```python
from build123d import *

# Parameters (mm, degrees)
F0_W      = 539.75
F0_H      = 53.975
F1_DEPTH  = 635
F2_W      = 482.854
F2_H      = 578.104
F3_DEPTH  = 25.4
F1_FACE_W = 539.75
F1_FACE_H = 635
F5_DEPTH  = 28.575


with BuildPart() as f1:
    # F0 (on Front) → F1 (new body)
    with BuildSketch(Plane.XZ):
        with Locations((269.875, 26.9875)):
            Rectangle(F0_W, F0_H)
    extrude(amount=-F1_DEPTH)

    # F2 (on face) → F3 (cut)
    with BuildSketch(Plane.XY.offset(53.975)):
        with Locations((269.875, 317.5)):
            Rectangle(F2_W, F2_H)
    extrude(amount=-F3_DEPTH, mode=Mode.SUBTRACT)


with BuildPart() as f5:
    # F1_face (on face) → F5 (new body)
    with BuildSketch(Plane(origin=(269.875, 317.5, 53.975), x_dir=(1, 0, 0), z_dir=(0, 0, 1))):
        Rectangle(F1_FACE_W, F1_FACE_H)
    extrude(amount=F5_DEPTH)


solid = f1.part
```
Source: CAD feature listing. Evaluate the final solid. Frame: model axes, mm. A direction names the side the tool comes from. Give positions to 0.01 mm unless a question says otherwise; leave off trailing zeros. Order: outer loops, then holes, each group sorted by start corner. A loop starts at its lowest first (then second) coordinate and runs counter-clockwise, first axis right, second up. Notation, with made-up numbers: (65.5, 77) -> (120.5, 77) arc R23 ccw to (120.5, 93) -> close; hole circle Ø4 at (38, 12). An arc over 180 degrees is marked (long way). Use a Markdown table: item, result.
Q1. Section C-C (x = 368). Return the cut outline in (y, z) (3 decimals).
A:
| item | result |
|---|---|
| outline | (0, 0) -> (635, 0) -> (635, 53.975) -> (606.552, 53.975) -> (606.552, 28.575) -> (28.448, 28.575) -> (28.448, 53.975) -> (0, 53.975) -> close |
Q2. Section B-B (z = 45.5). Return the cut outline in (x, y).
A:
| item | result |
|---|---|
| outline | (0, 0) -> (539.75, 0) -> (539.75, 635) -> (0, 635) -> close; hole (28.45, 28.45) -> (511.3, 28.45) -> (511.3, 606.55) -> (28.45, 606.55) -> close |
Q3. Pull-direction query (Y, two-part tool) for faces 3 (the face through (266, 606.552, 41)), 4 (the face through (0, 313, 27)), 5 (the face through (266, 0, 27)); classes: +Y half, -Y half, draft (parallel to the pull), parting line (faces both ways), or undercut.
A:
| item | result |
|---|---|
| face 3 | undercut |
| face 4 | draft |
| face 5 | -Y half |
Q4. First-contact query: P1, Ø5, axis at x = 267.5, z = 8.5, coming from the -Y side; P2, Ø4, axis at x = 195.5, y = 417.5, coming from the +Z side (3 decimals). Flat tips, straight axial feed; report the tip coordinate or a pass-through.
A:
| item | result |
|---|---|
| P1 | y = 0 |
| P2 | z = 28.575 |
Q5. Access query for faces 1 (the face through (266, 635, 27)), 2 (the face through (266, 28.448, 41)). Directions: +Z, -Z, +X, -X, +Y, -Y. A direction counts if a zero-diameter tool reaches every point of the face in a straight line with its end or side. Return the directions, or none.
A:
| item | result |
|---|---|
| face 1 | +Z, -Z, +X, -X, +Y |
| face 2 | +Z |
Q6. Section A-A (y = 242). Return the cut outline in (x, z) (3 decimals), and give its area (3 significant figures).
A:
| item | result |
|---|---|
| outline | (0, 0) -> (539.75, 0) -> (539.75, 53.975) -> (511.302, 53.975) -> (511.302, 28.575) -> (28.448, 28.575) -> (28.448, 53.975) -> (0, 53.975) -> close |
| area | 16,900 mm^2 |
Q7. Material intervals for line 1 (Y direction, x = 257.5, z = 35); line 2 (X direction, y = 463, z = 30); line 3 (Z direction, x = 217.5, y = 482) (3 decimals), sorted ascending. Write a range as [from, to].
A:
| item | result |
|---|---|
| line 1 | [0, 28.45], [606.55, 635] |
| line 2 | [0, 28.45], [511.3, 539.75] |
| line 3 | [0, 28.575] |
